Geometry: see drawing. Coordinates: mm, zero at the bounding-box minimum. A direction names the side the tool comes from. Coordinates: 2 decimals unless noted, no trailing zeros. Loops run counter-clockwise (first coordinate to the right, second up) from the corner with the lowest first, then second, coordinate; pieces in that order, holes last. Notation, with made-up numbers: (46, 53) - (64, 53) arc R29 ccw to (64, 77) - close; hole circle Ø8 at (39, -29.75). An arc over 180 degrees is marked (long way). Write each question's results on one line, items separated by ' | '. Start each with the question number.
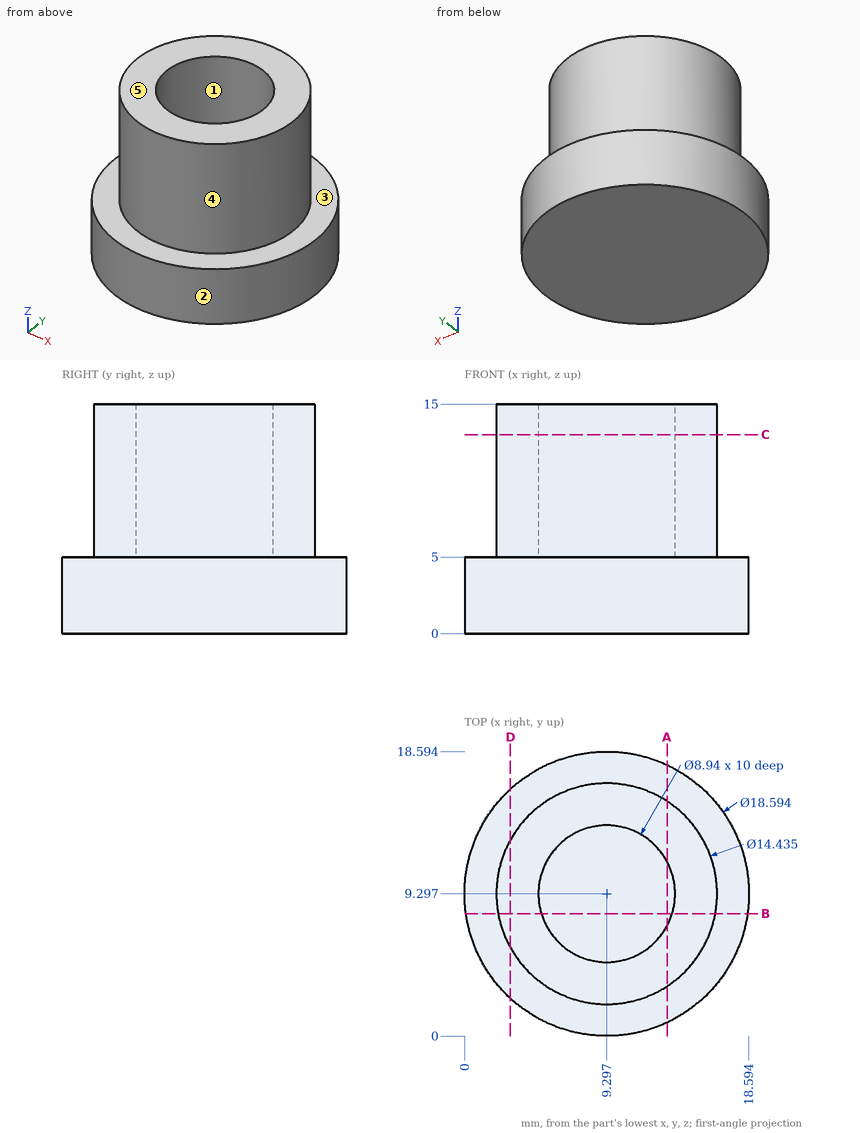
1) Material intervals for line 1 (Z direction, x = 17.5, y = 8.25); line 2 (Y direction, x = 11.5, z = 11.5); line 3 (Y direction, x = 10.5, z = 11.75), sorted ascending. Write a range as [from, to].
2) Section query B-B on y = 8. Output: boundary loops of the cut face in (x, z), and give its area (3 significant figures).
3) Pull-direction query (X, two-part tool) for the marked faces 1, 2 and 3; classes: released by +X, released by -X, zero draft, split by the parting line, or undercut.
4) Pin query (flat end, axial travel): pin 1 Ø1.5 at (x, y) = (11.5, 8.5) entering from +Z; pin 2 Ø3 at (y, z) = (5, 2.5) entering from -X; pin 3 Ø5 at (y, z) = (6, 2.5) entering from +X. Return the tip coordinate at first contact, or that it passes through.
5) Section query C-C on z = 13. Output: boundary loops of the cut face in (x, y) (1 decimal), and give its area (3 significant figures).
6) Section query A-A on x = 13.25. Output: boundary loops of the cut face in (y, z), and give its area (3 significant figures).
7) Section query D-D on x = 3. Output: boundary loops of the cut face in (y, z), and give its area (3 significant figures).
8) Access query for the marked faces 4 and 5. Directions: +Z, -Z, +X, -X, +Y, -Y. A direction counts if a zero-diameter tool reaches every point of the face in a straight line with its end or side. Return the directions, or none.
Returned:
1) line 1: z = [0, 5] | line 2: y = [2.42, 5.41], [13.19, 16.17] | line 3: y = [2.18, 4.99], [13.6, 16.41]
2) outline: (0.09, 0) - (18.5, 0) - (18.5, 5) - (16.4, 5) - (16.4, 15) - (13.57, 15) - (13.57, 5) - (5.02, 5) - (5.02, 15) - (2.2, 15) - (2.2, 5) - (0.09, 5) - close | area: 149 mm²
3) face 1: undercut | face 2: split by the parting line | face 3: zero draft
4) pin 1: stops at z = 5 | pin 2: stops at x = 0.43 | pin 3: stops at x = 18.56
5) outline: circle Ø14.4 at (9.3, 9.3); hole circle Ø8.9 at (9.3, 9.3) | area: 101 mm²
6) outline: (0.88, 0) - (17.71, 0) - (17.71, 5) - (15.34, 5) - (15.34, 15) - (11.38, 15) - (11.38, 5) - (7.21, 5) - (7.21, 15) - (3.26, 15) - (3.26, 5) - (0.88, 5) - close | area: 163 mm²
7) outline: (2.46, 0) - (16.14, 0) - (16.14, 5) - (12.82, 5) - (12.82, 15) - (5.77, 15) - (5.77, 5) - (2.46, 5) - close | area: 139 mm²
8) face 4: +Z | face 5: +Z, +X, -X, +Y, -Y
